Work out the finished part from the listing and answer in its coordinate system (mm). A direction names the side the tool comes from. Coordinates: 2 decimals unless noted, no trailing zeros. Write each loop counter-clockwise with the first axis right and the second up, starting at its lowest first coordinate (ties: lowest second). Pieces come first, ordered by that corner, then holes. Notation, with made-up numbers: (14.5, 13) - (20.5, 13) arc R11 ccw to (20.5, 32) - close; hole circle Ø9 at (20, -25). An arc over 180 degrees is marked (long way). Use CSV: the item, a comma, the result in double quotes. Start each with the question number.
from build123d import *

# Parameters (mm, degrees)
SKETCH_1_W      = 83
SKETCH_1_H      = 58
SKETCH_1_W_2    = 10.1
SKETCH_1_H_2    = 20.1
EXTRUDE_1_DEPTH = 2
SKETCH_2_W      = 83
SKETCH_2_H      = 30
EXTRUDE_2_DEPTH = 3


with BuildPart() as part:
    # 草图1 → 凸台-拉伸1 (new body)
    with BuildSketch(Plane.XY):
        with Locations((-26.149980732, -49.330690158)):
            Rectangle(SKETCH_1_W, SKETCH_1_H)
        with Locations((3.800019268, -35.380690158)):
            Rectangle(SKETCH_1_W_2, SKETCH_1_H_2, mode=Mode.SUBTRACT)
        with Locations((-56.099980732, -35.380690158)):
            Rectangle(SKETCH_1_W_2, SKETCH_1_H_2, mode=Mode.SUBTRACT)
    extrude(amount=EXTRUDE_1_DEPTH)

    # 草图2 → 凸台-拉伸2 (add)
    with BuildSketch(Plane(origin=(0, 0, 0), x_dir=(-1, 0, 0), z_dir=(0, 0, -1))):
        with Locations((26.149980732, -63.330690158)):
            Rectangle(SKETCH_2_W, SKETCH_2_H)
    extrude(amount=EXTRUDE_2_DEPTH)


solid = part.part
Item 1: A cutting plane is placed at C-C (x = -4.5). Determine the outline of the cut face in (y, z), then the cut area to 3 significant figures.
Item 2: A cutting plane is placed at D-D (y = -47). Determine the outline of the cut face in (x, z), then the cut area to 3 significant figures.
Item 3: Straight lines are drawn through the part: probe 1 along X at (y, z) = (-36, 0.35); probe 2 along Y at (x, z) = (-60, 0.55); probe 3 along Y at (x, z) = (11, -0.2). For each, find the intervals that lie inside material, in ascending order. Write a range as [from, to].
Item 4: Determine the mould class of faces 1 (the face through (-26, -78.331, 0)), 2 (the face through (-27, -34, 0)), 3 (the face through (-51.05, -36, 1)) for opening direction Y: +Y half, -Y half, draft (parallel to the pull), parting line (faces both ways), or undercut.
Item 5: Which of the six approach directions +Z, -Z, +X, -X, +Y, -Y give full straight-line access (tool end or side, diameter ignored) to faces 4 (the face through (-27, -49, 2)), 5 (the face through (-26, -48.331, -1)), 6 (the face through (8.85, -36, 1))?
Item 6: A cutting plane is placed at B-B (z = 0.8). Determine the outline of the cut face in (x, y).
Item 7: A cutting plane is placed at A-A (y = -38). Determine the outline of the cut face in (x, z), then the cut area to 3 significant figures.
Item 8: Each of these flat-tipped pins is pushed along its axis until it touches: pin 1 (8.5 mm diameter, centred on x = -13, y = -34.5, fed in from -Z); pin 2 (1.5 mm diameter, centred on x = -44.5, z = -1, fed in from +Y). Where does it stop, or does it pass through?
Calculated:
1,outline,"(-78.33, -3) - (-48.33, -3) - (-48.33, 0) - (-20.33, 0) - (-20.33, 2) - (-78.33, 2) - close"
1,area,"206 mm²"
2,outline,"(-67.65, 0) - (15.35, 0) - (15.35, 2) - (-67.65, 2) - close"
2,area,"166 mm²"
3,probe 1,"x = [-67.65, -61.15], [-51.05, -1.25], [8.85, 15.35]"
3,probe 2,"y = [-78.33, -45.43], [-25.33, -20.33]"
3,probe 3,"y = [-78.33, -48.33]"
4,face 1,"-Y half"
4,face 2,"draft"
4,face 3,"undercut"
5,face 4,"+Z, +X, -X, +Y, -Y"
5,face 5,"-Z, +X, -X, +Y"
5,face 6,"+Z, -Z"
6,outline,"(-67.65, -78.33) - (15.35, -78.33) - (15.35, -20.33) - (-67.65, -20.33) - close; hole (-61.15, -45.43) - (-51.05, -45.43) - (-51.05, -25.33) - (-61.15, -25.33) - close; hole (-1.25, -45.43) - (8.85, -45.43) - (8.85, -25.33) - (-1.25, -25.33) - close"
7,outline,"(-67.65, 0) - (-61.15, 0) - (-61.15, 2) - (-67.65, 2) - close; (-51.05, 0) - (-1.25, 0) - (-1.25, 2) - (-51.05, 2) - close; (8.85, 0) - (15.35, 0) - (15.35, 2) - (8.85, 2) - close"
7,area,"126 mm²"
8,pin 1,"stops at z = 0"
8,pin 2,"stops at y = -48.33"
